Verification items for the finished model (mm, model axes). Face numbers are marked on the shaded views. A direction names the side the tool comes from. Coordinates: 2 decimals unless noted, no trailing zeros. Write each loop counter-clockwise with the first axis right and the second up, starting at its lowest first coordinate (ties: lowest second). Pieces come first, ordered by that corner, then holes. Notation, with made-up numbers: M 23.25,-17 L 31.25,-17 A32 cw 31.25,13 Z; hole C 29,-38 d2. An arc over 180 degrees is marked long. One line per item, written item: value.
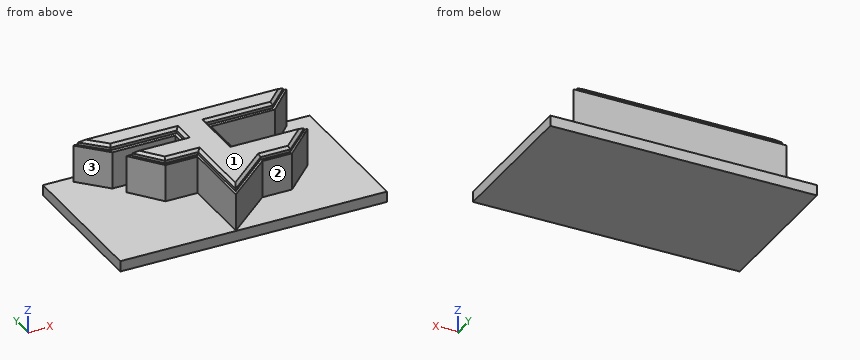
```python
from build123d import *

# Parameters (mm, degrees)
F1_DEPTH = 9
F3_DEPTH = 10
F4_SIZE  = 0.5
F5_W     = 50
F5_H     = 28.125
F6_DEPTH = 2


with BuildPart() as f1:
    # F0 (on Top) → F1 (new body)
    with BuildSketch(Plane.XY):
        Polygon((45.063734, 26.990574), (5.092878, 26.825527), (5.026509, 26.825527), (5.026509, 26.775939), (9.752492, 21.845225), (21.620436, 21.900864), (21.620436, 19.744122), (13.590824, 19.655766), (11.297298, 19.655766), (15.708311, 14.049002), (21.73431, 14.049002), (21.73431, 13.644104), (21.73431, 0.123029), (30.663192, 7.83794), (36.236674, 7.83794), (42.195871, 13.755384), (42.170566, 13.813944), (28.305346, 13.917539), (28.29141, 18.968888), (28.29141, 21.87437), (40.296681, 21.950597), (45.063985, 26.929848), align=None)
    extrude(amount=F1_DEPTH)

    # F2 (on Top) → F3 (join)
    with BuildSketch(Plane.XY):
        Polygon((44.290613, 26.706943), (5.77521, 26.568018), (9.783478, 22.559412), (22.173569, 22.559412), (22.173569, 19.259503), (12.177236, 19.259503), (15.873199, 14.606038), (22.135269, 14.606038), (22.135269, 0.990343), (30.599596, 8.363117), (36.172263, 8.363117), (41.38108, 13.437884), (27.75046, 13.437884), (27.75046, 22.559412), (40.209763, 22.559412), align=None)
    extrude(amount=F3_DEPTH)

    # F4
    f4_edges = [f1.edges().sort_by_distance(p)[0] for p in [
        (22.135269, 7.798191, 10),
        (26.367432, 4.67673, 10),
        (33.38593, 8.363117, 10),
        (38.776672, 10.900501, 10),
        (34.56577, 13.437884, 10),
        (27.75046, 17.998648, 10),
        (33.980112, 22.559412, 10),
        (42.250188, 24.633178, 10),
        (25.032912, 26.637481, 10),
        (7.779344, 24.563715, 10),
        (15.978524, 22.559412, 10),
        (22.173569, 20.909457, 10),
        (17.175402, 19.259503, 10),
        (14.025218, 16.932771, 10),
        (19.004234, 14.606038, 10),
    ]]
    chamfer(f4_edges, length=F4_SIZE)

    # F5 (on Top) → F6 (join)
    with BuildSketch(Plane.XY):
        with Locations((25, 14.0625)):
            Rectangle(F5_W, F5_H)
    extrude(amount=F6_DEPTH)


solid = f1.part
```
Item 1: Cross-section at C-C, the plane y = 6. Enter the section's corners in (x, z).
The answers:
outline: M 0,0 L 50,0 L 50,2 L 28.54,2 L 28.54,9 L 27.89,9 L 27.89,9.5 L 27.13,10 L 22.64,10 L 22.14,9.5 L 22.14,9 L 21.73,9 L 21.73,2 L 0,2 Z
Item 2: Go/stop test with flat-tipped pins: P1, Ø2.5, axis at x = 13, z = 6.5, coming from the +Y side; P2, Ø2, axis at x = 40.5, z = 1.5, coming from the -Y side; P3, Ø3, axis at x = 16, z = 4.5, coming from the -Y side; P4, Ø2, axis at x = 15, y = 5, coming from the +Z side. Record where each tip stops, or that it passes through.
The answers:
P1: stops at y = 26.86
P2: stops at y = 0
P3: stops at y = 14.05
P4: stops at z = 2
Item 3: Access from +Z, -Z, +X, -X, +Y, -Y to the whole of each face (thin tool, end or side, straight path). Record for the marked faces 1, 2 and 3.
The answers:
face 1: +Z, +X, -X, +Y, -Y
face 2: +Z, +X, -Y
face 3: +Z, -X, -Y
Item 4: Cross-section at B-B, the plane x = 23.5. Enter the section's corners in (y, z) (3 decimals).
The answers:
outline: M 0,0 L 28.125,0 L 28.125,2 L 26.902,2 L 26.902,9 L 26.632,9 L 26.632,9.5 L 26.132,10 L 2.842,10 L 2.179,9.5 L 2.179,9 L 1.649,9 L 1.649,2 L 0,2 Z
Item 5: Cross-section at A-A, the plane z = 4.5. Enter the section's corners in (x, y).
The answers:
outline: M 5.03,26.78 L 9.75,21.85 L 21.62,21.9 L 21.62,19.74 L 13.59,19.66 L 11.3,19.66 L 15.71,14.05 L 21.73,14.05 L 21.73,0.12 L 30.66,7.84 L 36.24,7.84 L 42.2,13.76 L 42.17,13.81 L 28.31,13.92 L 28.29,18.97 L 28.29,21.87 L 40.3,21.95 L 45.06,26.93 L 45.06,26.99 L 5.09,26.83 L 5.03,26.83 Z
Item 6: Scan lines: line 1 (Z direction, x = 37, y = 8.25); line 2 (X direction, y = 21.5, z = 6.75); line 3 (Y direction, x = 28.5, z = 3.5). Record each from-to range of solid material in increasing order.
The answers:
line 1: z = 0 to 2
line 2: x = 21.62 to 28.29
line 3: y = 5.97 to 13.92, 21.88 to 26.92
